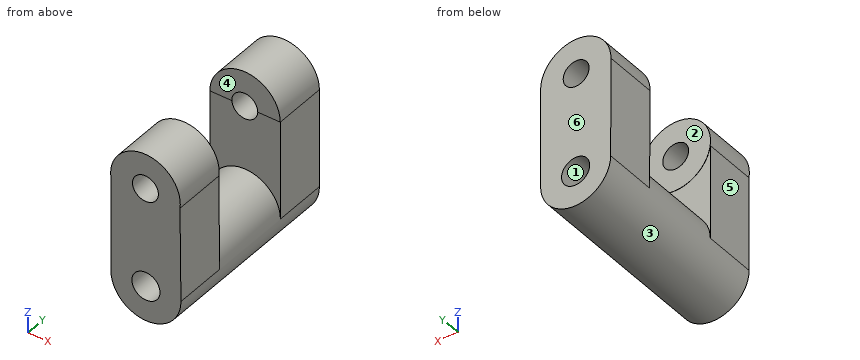
from build123d import *

# Parameters (mm, degrees)
F0_R      = 24.5736759636
F1_DEPTH  = 132.6354444027
F3_DEPTH  = 37.1311903
F5_DEPTH  = 37.3494811356
F6_R      = 24.4451738852
F7_DEPTH  = 37.2475758195
F9_DEPTH  = 37.4989584088
F10_R     = 9.0771573753
F11_DEPTH = 132.6364444027
F12_R     = 9.865321572
F13_DEPTH = 132.6364444027


with BuildPart() as f1:
    # F0 (on Front) → F1 (new body)
    with BuildSketch(Plane.XZ):
        with Locations((-8.2066878676, -21.1306065321)):
            Circle(F0_R)
    extrude(amount=-F1_DEPTH)

    # F2 (on face) → F3 (join)
    with BuildSketch(Plane.XZ):
        with BuildLine():
            ThreePointArc((-32.7796682644, -20.9457152509), (-32.7803638313, -21.1306065321), (-32.7796682644, -21.3154978133))
            Line((-32.7796682644, -21.3154978133), (-32.7796682644, -20.9457152509))
        make_face()
        with BuildLine():
            Line((-32.7796682644, 48.4050292678), (-32.7796682644, -20.9457152509))
            ThreePointArc((-32.7796682644, -20.9457152509), (-8.240472411, 3.4430462076), (16.3656912495, -20.8781488397))
            Line((16.3656912495, -20.8781488397), (15.6538728625, 48.4050292678))
            Line((15.6538728625, 48.4050292678), (-32.7796682644, 48.4050292678))
        make_face()
    extrude(amount=-F3_DEPTH)

    # F4 (on face) → F5 (join)
    with BuildSketch(Plane(origin=(0, 132.6354444027, 0), x_dir=(-1, 0, 0), z_dir=(0, 1, 0))):
        with BuildLine():
            Line((-16.3667459156, 48.1888727813), (-16.3667459156, -21.2397049542))
            ThreePointArc((-16.3667459156, -21.2397049542), (8.2016739749, 3.3337506723), (32.7801643053, -21.2296324502))
            Line((32.7801643053, -21.2296324502), (33.0599062145, 48.1888727813))
            Line((33.0599062145, 48.1888727813), (-16.3667459156, 48.1888727813))
        make_face()
    extrude(amount=-F5_DEPTH)

    # F6 (on face) → F7 (join)
    with BuildSketch(Plane.XZ):
        with Locations((-8.562897701, 48.4050292678)):
            Circle(F6_R)
    extrude(amount=-F7_DEPTH)

    # F8 (on face) → F9 (join)
    with BuildSketch(Plane(origin=(0, 132.6354444027, 0), x_dir=(-1, 0, 0), z_dir=(0, 1, 0))):
        with BuildLine():
            Line((-16.3667459156, 48.1888727813), (33.0599062145, 48.1888727813))
            ThreePointArc((33.0599062145, 48.1888727813), (8.3465801494, 72.9021988463), (-16.3667459156, 48.1888727813))
        make_face()
    extrude(amount=-F9_DEPTH)

    # F10 (on face) → F11 (cut, through all)
    with BuildSketch(Plane.XZ):
        with Locations((-8.562897701, 48.4050292678)):
            Circle(F10_R)
    extrude(amount=-F11_DEPTH, mode=Mode.SUBTRACT)

    # F12 (on face) → F13 (cut, through all)
    with BuildSketch(Plane.XZ):
        with Locations((-8.2066878676, -21.1306065321)):
            Circle(F12_R)
    extrude(amount=-F13_DEPTH, mode=Mode.SUBTRACT)


solid = f1.part
Input: part model. Units: mm. Frame: model coordinates. Face numbers are marked on the shaded views. A direction names the side the tool comes from. Give positions to 0.01 mm unless a question says otherwise; leave off trailing zeros. Write each loop counter-clockwise with the first axis right and the second up, starting at its lowest first coordinate (ties: lowest second). Pieces come first, ordered by that corner, then holes. Notation, with made-up numbers: (34, 12.5) -> (73, 12.5) arc R28 cw to (73, 32.5) -> close; hole circle Ø3 at (13, 11). An arc over 180 degrees is marked (long way). Use one line per item in the form item = value. Start each with the question number.
1) Draft query along Y for the marked faces 4, 5 and 6. Return one class per face: pulls with the +Y half, pulls with the -Y half, needs draft (parallel to the pull), parting line crosses it, or undercut.
2) Ray query, probe 1 along Y at (x, z) = (-8, 38); probe 2 along Y at (x, z) = (-10.5, 5.5); probe 3 along X at (y, z) = (26, 45.5). Return the intervals inside material, ascending. Write a range as from..to.
3) Set-up query: the marked faces 1, 2 and 3. Return all of +Z, -Z, +X, -X, +Y, -Y with unobstructed straight access to the full face (end or side cutting, diameter ignored); none if empty.
4) Section query D-D on z = 30.5. Return the cut outline in (x, y), then the cut area to 3 significant figures.
5) Section query B-B on x = -12. Return the cut outline in (y, z), then the cut area to 3 significant figures.
6) Section query A-A on z = 60. Return the cut outline in (x, y), then the cut area to 3 significant figures.
7) Section query C-C on y = 15. Return the cut outline in (x, z).
8) Pin query (flat end, axial travel): pin 1 (10 mm diameter, centred on x = 0, z = 6.5, fed in from -Y); pin 2 (18.5 mm diameter, centred on y = 17, z = 15.5, fed in from -X); pin 3 (4 mm diameter, centred on x = -7, y = 93, fed in from +Z); pin 4 (12 mm diameter, centred on x = -1, y = 90, fed in from -Z). Return the tip coordinate at first contact, or that it passes through.
Outcome:
q1.face_4 = undercut
q1.face_5 = needs draft
q1.face_6 = pulls with the +Y half
q2.probe_1 = 0..37.25, 95.29..132.64
q2.probe_2 = 0..37.13, 95.29..132.64
q2.probe_3 = -32.83..-17.16, 0.04..15.71
q3.face_1 = +Y, -Y
q3.face_2 = +Z, +X, -X
q3.face_3 = none
q4.outline = (-32.99, 95.29) -> (16.37, 95.29) -> (16.37, 132.64) -> (-32.99, 132.64) -> close; (-32.78, 0) -> (15.84, 0) -> (15.84, 37.13) -> (8.08, 37.13) -> (8.08, 37.25) -> (-25.21, 37.25) -> (-25.21, 37.13) -> (-32.78, 37.13) -> close
q4.area = 3,650 mm^2
q5.outline = (0, -45.41) -> (132.64, -45.41) -> (132.64, -30.24) -> (0, -30.24) -> close; (0, -12.02) -> (132.64, -12.02) -> (132.64, 40) -> (95.29, 40) -> (95.29, 3.15) -> (37.13, 3.15) -> (37.13, 24.2) -> (37.25, 24.2) -> (37.25, 40) -> (0, 40) -> close; (0, 56.81) -> (37.25, 56.81) -> (37.25, 72.61) -> (0, 72.61) -> close; (95.14, 56.81) -> (132.64, 56.81) -> (132.64, 72.63) -> (95.14, 72.63) -> close
q5.area = 7,950 mm^2
q6.outline = (-30.08, 0) -> (12.96, 0) -> (12.96, 37.25) -> (-30.08, 37.25) -> close; (-30.05, 95.14) -> (13.36, 95.14) -> (13.36, 132.64) -> (-30.05, 132.64) -> close
q6.area = 3,230 mm^2
q7.outline = (-32.78, -20.95) arc R24.57 ccw (long way) to (16.37, -20.88) -> (15.69, 45.31) arc R24.45 ccw (long way) to (-32.78, 45.07) -> close; hole circle Ø19.73 at (-8.21, -21.13); hole circle Ø18.15 at (-8.56, 48.41)
q8.pin_1 = 0
q8.pin_2 = -32.78
q8.pin_3 = 3.44
q8.pin_4 = -45.67
